```python
from build123d import *

# Parameters (mm, degrees)
F0_W     = 100
F0_H     = 50
F1_DEPTH = 2.5
F2_W     = 5
F2_H     = 5
F3_DEPTH = 40
F4_R     = 1
F5_DEPTH = 50.001


with BuildPart() as f1:
    # F0 (on Top) → F1 (new body)
    with BuildSketch(Plane.XY):
        with Locations((-1.152176, -27.418026)):
            Rectangle(F0_W, F0_H)
    extrude(amount=F1_DEPTH)

    # F2 (on face) → F3 (join)
    with BuildSketch(Plane.XY.offset(2.5)):
        with Locations((-48.652176, -4.918026)):
            Rectangle(F2_W, F2_H)
        with Locations((46.347824, -4.918026)):
            Rectangle(F2_W, F2_H)
        with Locations((46.347824, -49.918026)):
            Rectangle(F2_W, F2_H)
        with Locations((-48.652176, -49.918026)):
            Rectangle(F2_W, F2_H)
    extrude(amount=-F3_DEPTH)

    # F4 (on face) → F5 (cut, through all)
    with BuildSketch(Plane.XZ.offset(52.418026)):
        with Locations((46.347824, -32.5)):
            Circle(F4_R)
        with Locations((46.347824, -20.5)):
            Circle(F4_R)
        with Locations((46.347824, -8.5)):
            Circle(F4_R)
        with Locations((-48.652176, -8.5)):
            Circle(F4_R)
        with Locations((-48.652176, -20.5)):
            Circle(F4_R)
        with Locations((-48.652176, -32.5)):
            Circle(F4_R)
    extrude(amount=-F5_DEPTH, mode=Mode.SUBTRACT)


solid = f1.part
```
Can you work these out from the model? Positions are in its coordinate system, mm. A direction names the side the tool comes from. Round coordinates to 2 decimals unless told otherwise and drop trailing zeros. Order: outer loops, then holes, each group sorted by start corner. A loop starts at its lowest first (then second) coordinate and runs counter-clockwise, first axis right, second up. Notation, with made-up numbers: (87, 49) -> (101, 49) arc R22 ccw to (101, 59) -> close; hole circle Ø8 at (83, 0.25). An arc over 180 degrees is marked (long way). Return JSON: item names as keys, results as strings. Group by question number.
1. I need wall thicknesses on line 1 (Z direction, x = -40, y = -42). Which ranges of the line are inside material? Lowest first, please. Write a range as [from, to].
2. If we section it at D-D, the plane y = -13: Write out the boundary of the cut face in (x, z).
3. Will these pins go through, and if not, where does the flat tip stop? pin 1 (6 mm diameter, centred on x = 8, y = -46, fed in from -Z); pin 2 (2.5 mm diameter, centred on x = -48.65, z = -20.5, fed in from +Y).
4. If we section it at A-A, the plane z = -20.5: Count the separate pieces of the cut face and the enclosed holes in it, then the cut area to 3 significant figures.
5. If we section it at B-B, the plane z = -11.5: Write out the boundary of the cut face in (x, y), then the cut area to 3 significant figures.
6. If we section it at C-C, the plane x = 31: Write out the boundary of the cut face in (y, z), then the cut area to 3 significant figures.
7. We'd pull the mould along Y, two halves only. Please class faces 1 (the face through (46, -47.418, -18)), 2 (the face through (-51.152, -27.5, 0.2)): released by +Y, released by -Y, zero draft, split by the parting line, or undercut.
8. Which directions (+Z, -Z, +X, -X, +Y, -Y) give clear straight access to the entire face, cutting with the end or side of a thin tool? Please do faces 3 (the face through (-47.7, -50, -32.2)), 4 (the face through (43.848, -50, -18)), 5 (the face through (-49, -47.418, -18)).
Output values:
{
 "1": {"line 1": "[0, 2.5]"},
 "2": {"outline": "(-51.15, 0) -> (48.85, 0) -> (48.85, 2.5) -> (-51.15, 2.5) -> close"},
 "3": {"pin 1": "z = 0", "pin 2": "y = -2.42"},
 "4": {"separate pieces": "8", "enclosed holes": "0", "area": "60.0 mm²"},
 "5": {"outline": "(-51.15, -52.42) -> (-46.15, -52.42) -> (-46.15, -47.42) -> (-51.15, -47.42) -> close; (-51.15, -7.42) -> (-46.15, -7.42) -> (-46.15, -2.42) -> (-51.15, -2.42) -> close; (43.85, -52.42) -> (48.85, -52.42) -> (48.85, -47.42) -> (43.85, -47.42) -> close; (43.85, -7.42) -> (48.85, -7.42) -> (48.85, -2.42) -> (43.85, -2.42) -> close", "area": "100 mm²"},
 "6": {"outline": "(-52.42, 0) -> (-2.42, 0) -> (-2.42, 2.5) -> (-52.42, 2.5) -> close", "area": "125 mm²"},
 "7": {"face 1": "undercut", "face 2": "zero draft"},
 "8": {"face 3": "+Y, -Y", "face 4": "-Z, +Y, -Y", "face 5": "-Z, +X, -X"}
}
